```python
from build123d import *

# Parameters (mm, degrees)
F1_DEPTH = 100
F2_T     = -1
F4_DEPTH = 198


with BuildPart() as f1:
    # F0 (on Right) → F1 (new body, symmetric)
    with BuildSketch(Plane.YZ):
        Polygon((5.8090751991, 1.8115955126), (0, 1.8115955126), (-1.3203158755, 1.8115955126), (-1.3203158755, 0.5179099389), align=None)
        Polygon((-1.3203158755, 1.8115955126), (0, 1.8115955126), (5.8090751991, 1.8115955126), (0, 7.6206707116), (-19.7975447644, 7.6206707116), (-19.7975447644, -20.3238854808), (0, -20.3238854808), (0, -8.9974796865), (0, -3.1884044874), (-1.3203158755, -3.1884044874), (-1.3203158755, 0.5179099389), align=None)
        Polygon((5.8090751991, -3.1884044874), (0, -3.1884044874), (0, -8.9974796865), align=None)
    extrude(amount=F1_DEPTH, both=True)

    # F2
    f2_openings = [f1.faces().sort_by_distance(p)[0] for p in [
        (0, -9.898772, 7.620671),
    ]]
    offset(amount=F2_T, openings=f2_openings, kind=Kind.INTERSECTION)

    # F3 (on face) → F4 (join, through all)
    with BuildSketch(Plane.YZ.offset(-99)):
        Polygon((-1.4142135624, 7.6206707116), (-2.3203158755, 1.3527820438), (3.7518344093, 2.4546227399), align=None)
        Polygon((3.3948616367, -4.1884044874), (-2.3203158755, -4.1884044874), (-1, -8.5832661241), align=None)
    extrude(amount=F4_DEPTH)


solid = f1.part
```
The model under review builds one solid part; all positions refer to its coordinate system, in mm. A direction names the side the tool comes from. Give positions to 0.01 mm unless a question says otherwise; leave off trailing zeros. Write each loop counter-clockwise with the first axis right and the second up, starting at its lowest first coordinate (ties: lowest second). Pieces come first, ordered by that corner, then holes. Notation, with made-up numbers: M -8.75,-9.5 L 43.25,-9.5 A13 ccw 43.25,-5.5 Z; hole C -11,3 d6. An arc over 180 degrees is marked long. Write each question's results on one line, items separated by ' | '. Start each with the question number.
1. For probe 1 along X at (y, z) = (-13.5, 3.75); probe 2 along Y at (x, z) = (17, -9.5); probe 3 along Y at (x, z) = (-51, -8.5), list the stretches that pass through material, from the lowest coordinate up. Write a range as [from, to].
2. Mouldability with a two-part tool opening along Z and no side actions: class faces 1 (the flat face through (1, -19.798, -6)), 2 (the flat face through (1, 2, -3.188)), 3 (the flat face through (0, -1, 7.621)), 4 (the flat face through (-1.39, -1.67, -6.36)) as released by +Z, released by -Z, zero draft, split by the parting line, or undercut.
3. We need section A-A (z = -12.25). Write out the cut boundary in (x, y), and give its area (3 significant figures).
4. We need section B-B (x = -66.5). Write out the cut boundary in (y, z).
5. We need section C-C (y = -10.25). Write out the cut boundary in (x, z), and give its area (3 significant figures).
6. Insertion check: pin 1 Ø1.9 at (x, z) = (-32, -2) entering from +Y; pin 2 Ø12.5 at (x, z) = (-18.5, -14) entering from +Y; pin 3 Ø5.5 at (x, y) = (43.5, 3) entering from +Z. Each pin has a flat end and moves straight along its axis. Give the tip position at first contact, or say it passes through.
7. For faces 5 (the flat face through (-1.39, -1.86, 4.53)), 6 (the flat face through (1, -1.32, -1)), 7 (the flat face through (1, 0, -15)), 8 (the flat face through (1, -1, -14)), list the 3-axis set-ups (+Z, -Z, +X, -X, +Y, -Y) from which the entire face can be reached by the end or side of a thin tool; tool diameter is ignored.
Results found:
1) probe 1: x = [-100, -99], [99, 100] | probe 2: y = [-19.8, -18.8], [-1, 0] | probe 3: y = [-19.8, -18.8], [-1.03, 0.5]
2) face 1: zero draft | face 2: undercut | face 3: released by +Z | face 4: undercut
3) outline: M -100,-19.8 L 100,-19.8 L 100,0 L -100,0 Z; hole M -99,-18.8 L 99,-18.8 L 99,-1 L -99,-1 Z | area: 436 mm^2
4) outline: M -19.8,-20.32 L 0,-20.32 L 0,-9 L 5.81,-3.19 L -1.32,-3.19 L -1.32,0.52 L 5.81,1.81 L 0,7.62 L -1.41,7.62 L -2.32,1.35 L -2.32,-4.19 L -1,-8.58 L -1,-19.32 L -18.8,-19.32 L -18.8,7.62 L -19.8,7.62 Z
5) outline: M -100,-20.32 L 100,-20.32 L 100,7.62 L 99,7.62 L 99,-19.32 L -99,-19.32 L -99,7.62 L -100,7.62 Z | area: 254 mm^2
6) pin 1: stops at y = -1.32 | pin 2: stops at y = 1.25 | pin 3: stops at z = 7.37
7) face 5: +Z | face 6: +X, -X, +Y | face 7: -Z, +X, -X, +Y | face 8: none
